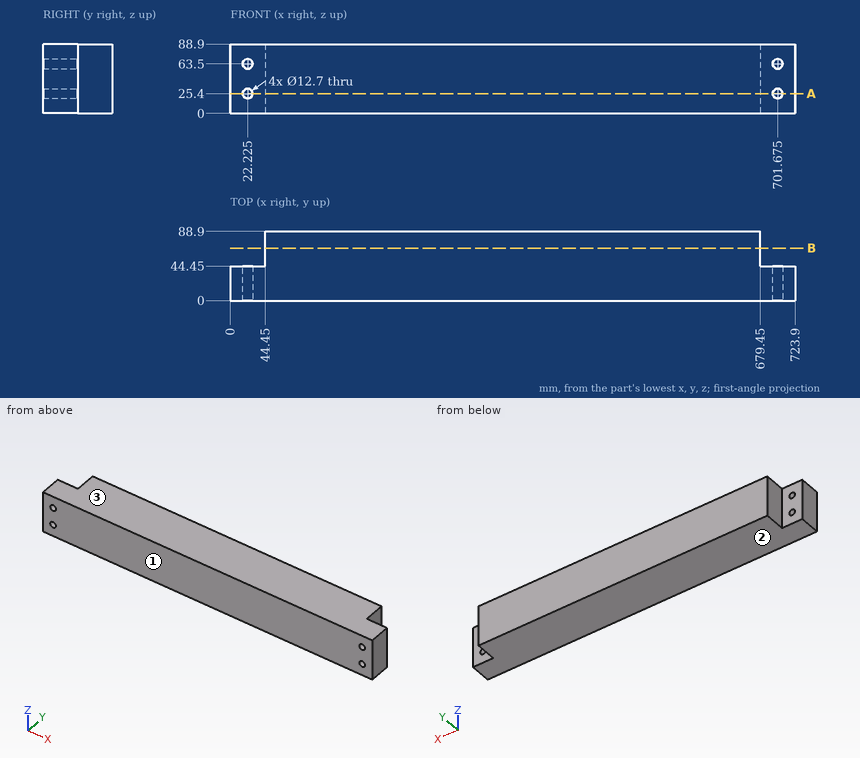
Print and shaded views of the part. All mm, measured from the part's lowest x, y and z. Give positions to 0.01 mm unless a question says otherwise; leave off trailing zeros. Write each loop counter-clockwise with the first axis right and the second up, starting at its lowest first coordinate (ties: lowest second). Pieces come first, ordered by that corner, then holes. Notation, with made-up numbers: (49, -26.5) - (63, -26.5) arc R13 cw to (63, -1.5) - close; hole circle Ø7 at (34.25, -18.5). An arc over 180 degrees is marked (long way). Put each result on its own line as item: value.
(1) Wall check: L1, parallel to X at y = 13, z = 25; L2, parallel to X at y = 65.5, z = 39.5. Give the ranges that are in metal, low to high.
Working result:
L1: 0 to 15.89, 28.56 to 695.34, 708.01 to 723.9
L2: 44.45 to 679.45
(2) Drop flat-ended pins along their axis: pin 1 Ø13.5 at (y, z) = (74, 66) entering from +X; pin 2 Ø22 at (y, z) = (66.5, 55.5) entering from -X; pin 3 Ø10 at (x, z) = (22.225, 63.5) entering from -Y. Give the stop position or say it passes through.
Working result:
pin 1: x = 679.45
pin 2: x = 44.45
pin 3: through
(3) Saw through at A-A (z = 25.4). List the corners of the cut face in (x, y) (3 decimals).
Working result:
outline: (0, 0) - (15.875, 0) - (15.875, 44.45) - (0, 44.45) - close; (28.575, 0) - (695.325, 0) - (695.325, 44.45) - (679.45, 44.45) - (679.45, 88.9) - (44.45, 88.9) - (44.45, 44.45) - (28.575, 44.45) - close; (708.025, 0) - (723.9, 0) - (723.9, 44.45) - (708.025, 44.45) - close
(4) Saw through at B-B (y = 67.5). List the corners of the cut face in (x, z), then the cut area to 3 significant figures.
Working result:
outline: (44.45, 0) - (679.45, 0) - (679.45, 88.9) - (44.45, 88.9) - close
area: 56,500 mm^2
(5) Pull direction Z, two halves, no side cores. Call the marked faces 1, 2 and 3: released by +Z, released by -Z, zero draft, split by the parting line, or undercut.
Working result:
face 1: zero draft
face 2: released by -Z
face 3: released by +Z
